The listing builds one solid part. Answer for the finished solid, in the listing's coordinates (mm). Give positions to 0.01 mm unless a question says otherwise; leave off trailing zeros. Loops run counter-clockwise (first coordinate to the right, second up) from the corner with the lowest first, then second, coordinate; pieces in that order, holes last. Notation, with made-up numbers: (39.5, -25) - (72.5, -25) arc R22 ccw to (72.5, -17) - close; hole circle Ø4 at (10.5, 49). An arc over 180 degrees is marked (long way). Answer in a Markdown table with one row per item. Add a question column.
```python
from build123d import *

# Parameters (mm, degrees)
CYLINDER002_R     = 0.75
CYLINDER002_DEPTH = 10
BOX005_W          = 12.8
BOX005_H          = 1
BOX005_DEPTH      = 0.75
CYLINDER001_R     = 1.8
CYLINDER001_DEPTH = 1.65


with BuildPart() as cylinder002:
    # Cylinder002 → Cylinder002 (new body)
    with BuildSketch(Plane(origin=(11.5, 6.7, 0), x_dir=(1, 0, 0), z_dir=(0, 0, 1))):
        Circle(CYLINDER002_R)
    extrude(amount=CYLINDER002_DEPTH)


with BuildPart() as sk1:
    # Box005 → Box005 (new body)
    with BuildSketch(Plane(origin=(2, 5.9, 0.9), x_dir=(1, 0, 0), z_dir=(0, 0, 1))):
        with Locations((6.4, 0.5)):
            Rectangle(BOX005_W, BOX005_H)
    extrude(amount=BOX005_DEPTH)


with BuildPart() as cut001:
    # Cylinder001 → Cylinder001 (new body)
    with BuildSketch(Plane(origin=(11.5, 6.7, 0), x_dir=(1, 0, 0), z_dir=(0, 0, 1))):
        Circle(CYLINDER001_R)
    extrude(amount=CYLINDER001_DEPTH)

    # Fusion001: union sk1
    add(sk1.part)

    # Cut001: cut Cylinder002
    add(cylinder002.part, mode=Mode.SUBTRACT)


solid = cut001.part
```
(1) A cutting plane is placed at B-B on y = 6.7. Determine the outline of the cut face in (x, z), plus the area to 3 significant figures.
(2) A cutting plane is placed at A-A on x = 11.5. Determine the outline of the cut face in (y, z), plus the area to 4 significant figures.
(3) The mould has two halves that part along Y. Classify faces 1 (the face through (10.905, 6.244, 0.813)), 2 (the face through (10, 6, 1.65)), 3 (the face through (11.266, 8.485, 0.813)): pulls with the +Y half, pulls with the -Y half, needs draft (parallel to the pull), parting line crosses it, or undercut.
(4) A cutting plane is placed at D-D on x = 6.5. Determine the outline of the cut face in (y, z), plus the area to 3 significant figures.
(5) A cutting plane is placed at C-C on z = 1.35. Determine the outline of the cut face in (x, y).
(6) Find the intervals of material crossed by line 1 along Y through (x, z) = (11.5, 0.3); line 2 along X through (y, z) = (6.7, 0.5); line 3 along X through (y, z) = (6.7, 1.25), in increasing order. Write a range as [from, to].
(7) Given pin 1 Ø1.7 at (x, y) = (11.5, 6.7) entering from -Z; pin 2 Ø2 at (x, y) = (8.5, 7) entering from -Z; pin 3 Ø0.6 at (x, z) = (7, 1.5) entering from +Y, each flat-ended and moving along its own axis, determine where each tip first touches the part or whether it passes through.
Evaluation:
| question | item | result |
|---|---|---|
| 1 | outline | (2, 0.9) - (9.7, 0.9) - (9.7, 0) - (10.75, 0) - (10.75, 1.65) - (2, 1.65) - close; (12.25, 0) - (13.3, 0) - (13.3, 0.9) - (14.8, 0.9) - (14.8, 1.65) - (12.25, 1.65) - close |
| 1 | area | 10.4 mm² |
| 2 | outline | (4.9, 0) - (5.95, 0) - (5.95, 1.65) - (4.9, 1.65) - close; (7.45, 0) - (8.5, 0) - (8.5, 1.65) - (7.45, 1.65) - close |
| 2 | area | 3.465 mm² |
| 3 | face 1 | undercut |
| 3 | face 2 | needs draft |
| 3 | face 3 | parting line crosses it |
| 4 | outline | (5.9, 0.9) - (6.9, 0.9) - (6.9, 1.65) - (5.9, 1.65) - close |
| 4 | area | 0.750 mm² |
| 5 | outline | (2, 5.9) - (9.89, 5.9) arc R1.8 ccw to (13.11, 5.9) - (14.8, 5.9) - (14.8, 6.9) - (13.29, 6.9) arc R1.8 ccw to (9.71, 6.9) - (2, 6.9) - close; hole circle Ø1.5 at (11.5, 6.7) |
| 6 | line 1 | y = [4.9, 5.95], [7.45, 8.5] |
| 6 | line 2 | x = [9.7, 10.75], [12.25, 13.3] |
| 6 | line 3 | x = [2, 10.75], [12.25, 14.8] |
| 7 | pin 1 | stops at z = 0 |
| 7 | pin 2 | stops at z = 0.9 |
| 7 | pin 3 | stops at y = 6.9 |
